from build123d import *

# Parameters (mm, degrees)
MAIN_DEPTH                         = 5.13
ASSEMBLY_SLOTS_REACH               = 7.13
SKETCH2_R                          = 1.5
SKETCH2_W                          = 5.13
SKETCH2_H                          = 58.88
SKETCH2_W_2                        = 58.88
SKETCH2_H_2                        = 5.13
LCD_AND_BLOCK_SLOT_REACH           = 7.13
SKETCH3_W                          = 40.4
SKETCH3_H                          = 98.1
SKETCH3_W_2                        = 44
SKETCH3_H_2                        = 44
LCD_SCREWHOLES_D                   = 3
LCD_SCREWHOLES_DEPTH               = 25.4
LCD_SCREWHOLES_TIP                 = 0.901290929
CORE_SCREWHOLES_PATTERN_COUNT      = 2
CORE_SCREWHOLES_PATTERN_PITCH      = 35
CORE_SCREWHOLES_PATTERN_COUNT_DIR2 = 2
CORE_SCREWHOLES_PATTERN_PITCH_DIR2 = 77
HINGE_SLOT_REACH                   = 7.13
SKETCH11_W                         = 22.5
SKETCH11_H                         = 44
LATCH_SLOT_REACH                   = 7.13
LID_THERMISTOR_HOLE_D              = 6.35
LID_THERMISTOR_HOLE_DEPTH          = 7.6
LID_THERMISTOR_HOLE_TIP            = 1.907732465


with BuildPart() as part:
    # Sketch1 → Main (new body)
    with BuildSketch(Plane(origin=(0, 0, 0), x_dir=(1, 0, 0), z_dir=(0, 1, 0))):
        with BuildLine():
            Line((-55.207201859, 101.249932113), (117.542798141, 101.249932113))
            ThreePointArc((117.542798141, 101.249932113), (126.523054262, 97.530188234), (130.242798141, 88.549932113))
            Line((130.242798141, 88.549932113), (130.242798141, -19.530067887))
            ThreePointArc((130.242798141, -19.530067887), (126.523054262, -28.510324008), (117.542798141, -32.230067887))
            Line((117.542798141, -32.230067887), (-55.207201859, -32.230067887))
            ThreePointArc((-55.207201859, -32.230067887), (-64.18745798, -28.510324008), (-67.907201859, -19.530067887))
            Line((-67.907201859, -19.530067887), (-67.907201859, 88.549932113))
            ThreePointArc((-67.907201859, 88.549932113), (-64.18745798, 97.530188234), (-55.207201859, 101.249932113))
        make_face()
    extrude(amount=MAIN_DEPTH)

    # Sketch2 → Assembly slots (cut, up to next)
    with BuildSketch(Plane(origin=(0, 5.13, 0), x_dir=(1, 0, 0), z_dir=(0, 1, 0)), mode=Mode.PRIVATE) as assembly_slots_sk1:
        with Locations((-28.272201859, 91.689932113)):
            Circle(SKETCH2_R)
    assembly_slots_tool1 = extrude(assembly_slots_sk1.sketch, amount=-ASSEMBLY_SLOTS_REACH, mode=Mode.PRIVATE) & part.part
    add(assembly_slots_tool1.solids().sort_by_distance((-28.272202, 5.13, -91.689932))[0], mode=Mode.SUBTRACT)
    # Sketch2 → Assembly slots (cut, up to next)
    with BuildSketch(Plane(origin=(0, 5.13, 0), x_dir=(1, 0, 0), z_dir=(0, 1, 0)), mode=Mode.PRIVATE) as assembly_slots_sk2:
        with Locations((90.607798141, 91.689932113)):
            Circle(SKETCH2_R)
    assembly_slots_tool2 = extrude(assembly_slots_sk2.sketch, amount=-ASSEMBLY_SLOTS_REACH, mode=Mode.PRIVATE) & part.part
    add(assembly_slots_tool2.solids().sort_by_distance((90.607798, 5.13, -91.689932))[0], mode=Mode.SUBTRACT)
    # Sketch2 → Assembly slots (cut, up to next)
    with BuildSketch(Plane(origin=(0, 5.13, 0), x_dir=(1, 0, 0), z_dir=(0, 1, 0)), mode=Mode.PRIVATE) as assembly_slots_sk3:
        with Locations((-58.347201859, -14.930067887)):
            Circle(SKETCH2_R)
    assembly_slots_tool3 = extrude(assembly_slots_sk3.sketch, amount=-ASSEMBLY_SLOTS_REACH, mode=Mode.PRIVATE) & part.part
    add(assembly_slots_tool3.solids().sort_by_distance((-58.347202, 5.13, 14.930068))[0], mode=Mode.SUBTRACT)
    # Sketch2 → Assembly slots (cut, up to next)
    with BuildSketch(Plane(origin=(0, 5.13, 0), x_dir=(1, 0, 0), z_dir=(0, 1, 0)), mode=Mode.PRIVATE) as assembly_slots_sk4:
        with Locations((-58.347201859, 83.949932113)):
            Circle(SKETCH2_R)
    assembly_slots_tool4 = extrude(assembly_slots_sk4.sketch, amount=-ASSEMBLY_SLOTS_REACH, mode=Mode.PRIVATE) & part.part
    add(assembly_slots_tool4.solids().sort_by_distance((-58.347202, 5.13, -83.949932))[0], mode=Mode.SUBTRACT)
    # Sketch2 → Assembly slots (cut, up to next)
    with BuildSketch(Plane(origin=(0, 5.13, 0), x_dir=(1, 0, 0), z_dir=(0, 1, 0)), mode=Mode.PRIVATE) as assembly_slots_sk5:
        with Locations((120.682798141, 83.949932113)):
            Circle(SKETCH2_R)
    assembly_slots_tool5 = extrude(assembly_slots_sk5.sketch, amount=-ASSEMBLY_SLOTS_REACH, mode=Mode.PRIVATE) & part.part
    add(assembly_slots_tool5.solids().sort_by_distance((120.682798, 5.13, -83.949932))[0], mode=Mode.SUBTRACT)
    # Sketch2 → Assembly slots (cut, up to next)
    with BuildSketch(Plane(origin=(0, 5.13, 0), x_dir=(1, 0, 0), z_dir=(0, 1, 0)), mode=Mode.PRIVATE) as assembly_slots_sk6:
        with Locations((120.682798141, -14.930067887)):
            Circle(SKETCH2_R)
    assembly_slots_tool6 = extrude(assembly_slots_sk6.sketch, amount=-ASSEMBLY_SLOTS_REACH, mode=Mode.PRIVATE) & part.part
    add(assembly_slots_tool6.solids().sort_by_distance((120.682798, 5.13, 14.930068))[0], mode=Mode.SUBTRACT)
    # Sketch2 → Assembly slots (cut, up to next)
    with BuildSketch(Plane(origin=(0, 5.13, 0), x_dir=(1, 0, 0), z_dir=(0, 1, 0)), mode=Mode.PRIVATE) as assembly_slots_sk7:
        with Locations((90.607798141, -22.670067887)):
            Circle(SKETCH2_R)
    assembly_slots_tool7 = extrude(assembly_slots_sk7.sketch, amount=-ASSEMBLY_SLOTS_REACH, mode=Mode.PRIVATE) & part.part
    add(assembly_slots_tool7.solids().sort_by_distance((90.607798, 5.13, 22.670068))[0], mode=Mode.SUBTRACT)
    # Sketch2 → Assembly slots (cut, up to next)
    with BuildSketch(Plane(origin=(0, 5.13, 0), x_dir=(1, 0, 0), z_dir=(0, 1, 0)), mode=Mode.PRIVATE) as assembly_slots_sk8:
        with Locations((-28.272201859, -22.670067887)):
            Circle(SKETCH2_R)
    assembly_slots_tool8 = extrude(assembly_slots_sk8.sketch, amount=-ASSEMBLY_SLOTS_REACH, mode=Mode.PRIVATE) & part.part
    add(assembly_slots_tool8.solids().sort_by_distance((-28.272202, 5.13, 22.670068))[0], mode=Mode.SUBTRACT)
    # Sketch2 → Assembly slots (cut, up to next)
    with BuildSketch(Plane(origin=(0, 5.13, 0), x_dir=(1, 0, 0), z_dir=(0, 1, 0)), mode=Mode.PRIVATE) as assembly_slots_sk9:
        with Locations((-58.342201859, 34.509932113)):
            Rectangle(SKETCH2_W, SKETCH2_H)
    assembly_slots_tool9 = extrude(assembly_slots_sk9.sketch, amount=-ASSEMBLY_SLOTS_REACH, mode=Mode.PRIVATE) & part.part
    add(assembly_slots_tool9.solids().sort_by_distance((-58.342202, 5.13, -34.509932))[0], mode=Mode.SUBTRACT)
    # Sketch2 → Assembly slots (cut, up to next)
    with BuildSketch(Plane(origin=(0, 5.13, 0), x_dir=(1, 0, 0), z_dir=(0, 1, 0)), mode=Mode.PRIVATE) as assembly_slots_sk10:
        with Locations((31.167798141, 91.684932113)):
            Rectangle(SKETCH2_W_2, SKETCH2_H_2)
    assembly_slots_tool10 = extrude(assembly_slots_sk10.sketch, amount=-ASSEMBLY_SLOTS_REACH, mode=Mode.PRIVATE) & part.part
    add(assembly_slots_tool10.solids().sort_by_distance((31.167798, 5.13, -91.684932))[0], mode=Mode.SUBTRACT)
    # Sketch2 → Assembly slots (cut, up to next)
    with BuildSketch(Plane(origin=(0, 5.13, 0), x_dir=(1, 0, 0), z_dir=(0, 1, 0)), mode=Mode.PRIVATE) as assembly_slots_sk11:
        with Locations((120.677798141, 34.509932113)):
            Rectangle(SKETCH2_W, SKETCH2_H)
    assembly_slots_tool11 = extrude(assembly_slots_sk11.sketch, amount=-ASSEMBLY_SLOTS_REACH, mode=Mode.PRIVATE) & part.part
    add(assembly_slots_tool11.solids().sort_by_distance((120.677798, 5.13, -34.509932))[0], mode=Mode.SUBTRACT)
    # Sketch2 → Assembly slots (cut, up to next)
    with BuildSketch(Plane(origin=(0, 5.13, 0), x_dir=(1, 0, 0), z_dir=(0, 1, 0)), mode=Mode.PRIVATE) as assembly_slots_sk12:
        with Locations((31.167798141, -22.665067887)):
            Rectangle(SKETCH2_W_2, SKETCH2_H_2)
    assembly_slots_tool12 = extrude(assembly_slots_sk12.sketch, amount=-ASSEMBLY_SLOTS_REACH, mode=Mode.PRIVATE) & part.part
    add(assembly_slots_tool12.solids().sort_by_distance((31.167798, 5.13, 22.665068))[0], mode=Mode.SUBTRACT)

    # Sketch3 → LCD and Block slot (cut, up to next)
    with BuildSketch(Plane.XZ, mode=Mode.PRIVATE) as lcd_and_block_slot_sk1:
        with Locations((-17.707201859, -34.509932113)):
            Rectangle(SKETCH3_W, SKETCH3_H)
    lcd_and_block_slot_tool1 = extrude(lcd_and_block_slot_sk1.sketch, amount=-LCD_AND_BLOCK_SLOT_REACH, mode=Mode.PRIVATE) & part.part
    add(lcd_and_block_slot_tool1.solids().sort_by_distance((-17.707202, 0, -34.509932))[0], mode=Mode.SUBTRACT)
    # Sketch3 → LCD and Block slot (cut, up to next)
    with BuildSketch(Plane.XZ, mode=Mode.PRIVATE) as lcd_and_block_slot_sk2:
        with Locations((63.742798141, -34.509932113)):
            Rectangle(SKETCH3_W_2, SKETCH3_H_2)
    lcd_and_block_slot_tool2 = extrude(lcd_and_block_slot_sk2.sketch, amount=-LCD_AND_BLOCK_SLOT_REACH, mode=Mode.PRIVATE) & part.part
    add(lcd_and_block_slot_tool2.solids().sort_by_distance((63.742798, 0, -34.509932))[0], mode=Mode.SUBTRACT)

    # LCD screwholes
    with Locations(Plane(origin=(0, 5.13, 0), x_dir=(-1, 0, 0), z_dir=(0, 1, 0))):
        with Locations((45.557201859, 11.990067887), (-9.442798141, 11.990067887), (45.557201859, -81.009932113), (-9.442798141, -81.009932113)):
            Hole(LCD_SCREWHOLES_D / 2, depth=LCD_SCREWHOLES_DEPTH)
            with Locations((0, 0, -(LCD_SCREWHOLES_DEPTH + LCD_SCREWHOLES_TIP / 2))):  # 118° drill point
                Cone(0, LCD_SCREWHOLES_D / 2, LCD_SCREWHOLES_TIP, mode=Mode.SUBTRACT)

    # Sketch8 → Core screwholes (revolve, cut)
    with BuildSketch(Plane(origin=(46.427392408, 5.13, -73.009932113), x_dir=(0, 0, 1), z_dir=(1, 0, 0))):
        Polygon((0, 0), (0, 26.301290929), (1.5, 25.4), (1.5, 0), align=None)
    core_screwholes = revolve(axis=Axis((46.427392408, 11.48, -73.009932113), (0, -1, 0)), mode=Mode.SUBTRACT)

    # Core screwholes pattern: Core screwholes 2 × 2
    with Locations(*[(i * CORE_SCREWHOLES_PATTERN_PITCH, 0, j * CORE_SCREWHOLES_PATTERN_PITCH_DIR2) for i in range(CORE_SCREWHOLES_PATTERN_COUNT) for j in range(CORE_SCREWHOLES_PATTERN_COUNT_DIR2) if (i, j) != (0, 0)]):
        add(core_screwholes, mode=Mode.SUBTRACT)

    # Sketch11 → Hinge slot (cut, up to next)
    with BuildSketch(Plane(origin=(0, 5.13, 0), x_dir=(1, 0, 0), z_dir=(0, 1, 0)), mode=Mode.PRIVATE) as hinge_slot_sk1:
        with Locations((106.874365391, 34.509932113)):
            Rectangle(SKETCH11_W, SKETCH11_H)
    hinge_slot_tool1 = extrude(hinge_slot_sk1.sketch, amount=-HINGE_SLOT_REACH, mode=Mode.PRIVATE) & part.part
    add(hinge_slot_tool1.solids().sort_by_distance((106.874365, 5.13, -34.509932))[0], mode=Mode.SUBTRACT)

    # Sketch13 → Latch Slot (cut, up to next)
    with BuildSketch(Plane(origin=(0, 5.13, 0), x_dir=(1, 0, 0), z_dir=(0, 1, 0)), mode=Mode.PRIVATE) as latch_slot_sk1:
        with BuildLine():
            Line((26.626560662, 48.479932113), (31.326560662, 48.479932113))
            ThreePointArc((31.326560662, 48.479932113), (32.033667443, 48.187038894), (32.326560662, 47.479932113))
            Line((32.326560662, 47.479932113), (32.326560662, 21.539932113))
            ThreePointArc((32.326560662, 21.539932113), (32.033667443, 20.832825332), (31.326560662, 20.539932113))
            Line((31.326560662, 20.539932113), (26.626560662, 20.539932113))
            ThreePointArc((26.626560662, 20.539932113), (25.919453881, 20.832825332), (25.626560662, 21.539932113))
            Line((25.626560662, 21.539932113), (25.626560662, 47.479932113))
            ThreePointArc((25.626560662, 47.479932113), (25.919453881, 48.187038894), (26.626560662, 48.479932113))
        make_face()
    latch_slot_tool1 = extrude(latch_slot_sk1.sketch, amount=-LATCH_SLOT_REACH, mode=Mode.PRIVATE) & part.part
    add(latch_slot_tool1.solids().sort_by_distance((28.976561, 5.13, -34.509932))[0], mode=Mode.SUBTRACT)

    # Lid thermistor hole
    with Locations(Plane(origin=(0, 5.13, 0), x_dir=(-1, 0, 0), z_dir=(0, 1, 0))):
        with Locations((-101.47244154, -70.602615051)):
            Hole(LID_THERMISTOR_HOLE_D / 2, depth=LID_THERMISTOR_HOLE_DEPTH)
            with Locations((0, 0, -(LID_THERMISTOR_HOLE_DEPTH + LID_THERMISTOR_HOLE_TIP / 2))):  # 118° drill point
                Cone(0, LID_THERMISTOR_HOLE_D / 2, LID_THERMISTOR_HOLE_TIP, mode=Mode.SUBTRACT)


solid = part.part
Model file for the job. Use its own axes, mm. A direction names the side the tool comes from. Give positions to 0.01 mm unless a question says otherwise; leave off trailing zeros. Order: outer loops, then holes, each group sorted by start corner. A loop starts at its lowest first (then second) coordinate and runs counter-clockwise, first axis right, second up. Notation, with made-up numbers: (21, 33) -> (77, 33) arc R22 cw to (77, 50) -> close; hole circle Ø4 at (-11.5, -7). An arc over 180 degrees is marked (long way). Use CSV: the item, a comma, the result in double quotes.
1. Band-saw the part on A-A, the plane x = -9.5. Give the cut face in (y, z), then the cut area to 3 significant figures.
Outcome:
outline,"(0, -101.25) -> (5.13, -101.25) -> (5.13, -83.56) -> (0, -83.56) -> close; (0, 14.54) -> (5.13, 14.54) -> (5.13, 32.23) -> (0, 32.23) -> close"
area,"181 mm²"
2. Drop a flat-ended pin along its axis: pin 1 (2.5 mm diameter, centred on x = -58.5, y = 2, fed in from -Z). Give the stop position or say it passes through.
Outcome:
pin 1,"z = -101.08"
3. Band-saw the part on C-C, the plane x = 73. Give the cut face in (y, z), then the cut area to 3 significant figures.
Outcome:
outline,"(0, -101.25) -> (5.13, -101.25) -> (5.13, -56.51) -> (0, -56.51) -> close; (0, -12.51) -> (5.13, -12.51) -> (5.13, 32.23) -> (0, 32.23) -> close"
area,"459 mm²"
4. Drill centre lines: line 1 along Z through (x, y) = (81.5, 0.3); line 2 along Z through (x, y) = (12, 2.2); line 3 along X through (y, z) = (3.9, -55.5). Where is each one in solid material? Low to high. Write a range as from..to.
Outcome:
line 1,"-101.25..-74.51, -71.51..-56.51, -12.51..2.49, 5.49..32.23"
line 2,"-101.25..-94.25, -89.12..20.1, 25.23..32.23"
line 3,"-67.91..-60.91, -55.78..-37.91, 2.49..41.74, 85.74..95.62, 123.24..130.24"
5. Band-saw the part on B-B, the plane z = -34.5. Give the cut face in (x, y), then the cut area to 3 significant figures.
Outcome:
outline,"(-67.91, 0) -> (-60.91, 0) -> (-60.91, 5.13) -> (-67.91, 5.13) -> close; (-55.78, 0) -> (-37.91, 0) -> (-37.91, 5.13) -> (-55.78, 5.13) -> close; (2.49, 0) -> (25.63, 0) -> (25.63, 5.13) -> (2.49, 5.13) -> close; (32.33, 0) -> (41.74, 0) -> (41.74, 5.13) -> (32.33, 5.13) -> close; (85.74, 0) -> (95.62, 0) -> (95.62, 5.13) -> (85.74, 5.13) -> close; (123.24, 0) -> (130.24, 0) -> (130.24, 5.13) -> (123.24, 5.13) -> close"
area,"381 mm²"
6. 3-axis set-ups, long thin cutter, end or side, ignore diameter. For faces 1 (the flat face through (41.743, 3, -35)), 2 (the flat face through (33, 0, -35)): which of +Z, -Z, +X, -X, +Y, -Y reach the whole face in a straight line?
Outcome:
face 1,"+Y, -Y"
face 2,"+Z, -Z, +X, -X, -Y"
7. Mould opens along Z. For faces 3 (the flat face through (130.243, 3, -35)), 4 (the cylindrical face through (98.95, 2.53, -72.53)), 5 (the cylindrical face through (126.62, 2.53, 28.41)) say: +Z half, -Z half, draft (parallel to the pull), parting line (faces both ways), or undercut.
Outcome:
face 3,"draft"
face 4,"undercut"
face 5,"+Z half"
8. Band-saw the part on D-D, the plane y = 2.05. Count the separate pieces of the cut face and the enclosed holes in it, then the cut area to 3 significant figures.
Outcome:
separate pieces,"1"
enclosed holes,"24"
area,"17,900 mm²"
